Verification items for the finished model (mm, model axes). Face numbers are marked on the shaded views. A direction names the side the tool comes from. Give positions to 0.01 mm unless a question says otherwise; leave off trailing zeros. Loops run counter-clockwise (first coordinate to the right, second up) from the corner with the lowest first, then second, coordinate; pieces in that order, holes last. Notation, with made-up numbers: M 69.25,-26 L 92.25,-26 A29 ccw 92.25,-5 Z; hole C 83.25,-38 d6. An arc over 180 degrees is marked long. Put each result on its own line as item: value. Start each with the question number.
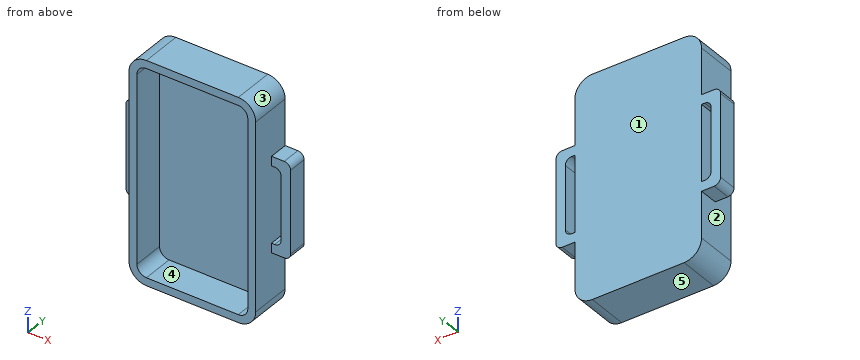
from build123d import *

# Parameters (mm, degrees)
F1_DEPTH = 3
F2_DEPTH = 13
F3_DEPTH = 6


with BuildPart() as f1:
    # F0 (on Front) → F1 (new body)
    with BuildSketch(Plane.XZ):
        with BuildLine():
            Line((-14.5, -32.5), (14.5, -32.5))
            ThreePointArc((14.5, -32.5), (16.62132, -31.62132), (17.5, -29.5))
            Line((17.5, -29.5), (17.5, 29.5))
            ThreePointArc((17.5, 29.5), (16.62132, 31.62132), (14.5, 32.5))
            Line((14.5, 32.5), (-14.5, 32.5))
            ThreePointArc((-14.5, 32.5), (-16.62132, 31.62132), (-17.5, 29.5))
            Line((-17.5, 29.5), (-17.5, -29.5))
            ThreePointArc((-17.5, -29.5), (-16.62132, -31.62132), (-14.5, -32.5))
        make_face()
    extrude(amount=F1_DEPTH)

    # F0 (on Front) → F2 (join)
    with BuildSketch(Plane.XZ):
        with BuildLine():
            Line((14.5, 35), (-14.5, 35))
            ThreePointArc((-14.5, 35), (-18.389087, 33.389087), (-20, 29.5))
            Line((-20, 29.5), (-20, 15))
            Line((-20, 15), (-20, 12))
            Line((-20, 12), (-20, -12))
            Line((-20, -12), (-20, -15))
            Line((-20, -15), (-20, -29.5))
            ThreePointArc((-20, -29.5), (-18.389087, -33.389087), (-14.5, -35))
            Line((-14.5, -35), (14.5, -35))
            ThreePointArc((14.5, -35), (18.389087, -33.389087), (20, -29.5))
            Line((20, -29.5), (20, -15))
            Line((20, -15), (20, -12))
            Line((20, -12), (20, 12))
            Line((20, 12), (20, 15))
            Line((20, 15), (20, 29.5))
            ThreePointArc((20, 29.5), (18.389087, 33.389087), (14.5, 35))
        make_face()
        with BuildLine():
            ThreePointArc((17.5, -29.5), (16.62132, -31.62132), (14.5, -32.5))
            Line((14.5, -32.5), (-14.5, -32.5))
            ThreePointArc((-14.5, -32.5), (-16.62132, -31.62132), (-17.5, -29.5))
            Line((-17.5, -29.5), (-17.5, 29.5))
            ThreePointArc((-17.5, 29.5), (-16.62132, 31.62132), (-14.5, 32.5))
            Line((-14.5, 32.5), (14.5, 32.5))
            ThreePointArc((14.5, 32.5), (16.62132, 31.62132), (17.5, 29.5))
            Line((17.5, 29.5), (17.5, -29.5))
        make_face(mode=Mode.SUBTRACT)
    extrude(amount=F2_DEPTH)

    # F0 (on Front) → F3 (join)
    with BuildSketch(Plane.XZ):
        with BuildLine():
            Line((-20, 12), (-20, 15))
            Line((-20, 15), (-24, 15))
            ThreePointArc((-24, 15), (-25.414214, 14.414214), (-26, 13))
            Line((-26, 13), (-26, -13))
            ThreePointArc((-26, -13), (-25.414214, -14.414214), (-24, -15))
            Line((-24, -15), (-20, -15))
            Line((-20, -15), (-20, -12))
            Line((-20, -12), (-21, -12))
            ThreePointArc((-21, -12), (-22.414214, -11.414214), (-23, -10))
            Line((-23, -10), (-23, 10))
            ThreePointArc((-23, 10), (-22.414214, 11.414214), (-21, 12))
            Line((-21, 12), (-20, 12))
        make_face()
        with BuildLine():
            Line((24, 15), (20, 15))
            Line((20, 15), (20, 12))
            Line((20, 12), (21, 12))
            ThreePointArc((21, 12), (22.414214, 11.414214), (23, 10))
            Line((23, 10), (23, -10))
            ThreePointArc((23, -10), (22.414214, -11.414214), (21, -12))
            Line((21, -12), (20, -12))
            Line((20, -12), (20, -15))
            Line((20, -15), (24, -15))
            ThreePointArc((24, -15), (25.414214, -14.414214), (26, -13))
            Line((26, -13), (26, 13))
            ThreePointArc((26, 13), (25.414214, 14.414214), (24, 15))
        make_face()
    extrude(amount=F3_DEPTH)


solid = f1.part
Q1. Cross-section at B-B, the plane y = -10. Record the boundary of the cut face in (x, z).
Q2. Go/stop test with flat-tipped pins: pin 1 (0.5 mm diameter, centred on x = 20.5, y = -3, fed in from +Z); pin 2 (1 mm diameter, centred on y = -4.5, z = -17.5, fed in from +X); pin 3 (3 mm diameter, centred on x = 22.5, z = -2.5, fed in from -Y); pin 4 (5 mm diameter, centred on x = -21.5, z = -2.5, fed in from -Y). Record where each tip stops, or that it passes through.
Q3. Cross-section at C-C, the plane x = 4. Record the boundary of the cut face in (y, z), then the cut area to 3 significant figures.
Q4. Cross-section at D-D, the plane z = 17. Record the boundary of the cut face in (x, y).
Q5. Cross-section at A-A, the plane z = 4. Record the boundary of the cut face in (x, y), then the cut area to 3 significant figures.
Q6. Scan lines: L1, parallel to X at y = -1, z = -1; L2, parallel to Z at x = -9.5, y = -3.5; L3, parallel to X at y = -10.25, z = -12. Record each from-to range of solid material in increasing order.
Q7. Release check for a two-part mould opening along Z. For the marked faces 3, 4 and 5 record: pulls with the +Z half, pulls with the -Z half, needs draft (parallel to the pull), parting line crosses it, or undercut.
Q8. Set-up check for the marked faces 1 and 2: record each of +Z, -Z, +X, -X, +Y, -Y from which the full face is reachable in a straight line by a thin tool's end or side.
Ans:
1. outline: M -20,-29.5 A5.5 ccw -14.5,-35 L 14.5,-35 A5.5 ccw 20,-29.5 L 20,29.5 A5.5 ccw 14.5,35 L -14.5,35 A5.5 ccw -20,29.5 Z; hole M -17.5,-29.5 A3 ccw -14.5,-32.5 L 14.5,-32.5 A3 ccw 17.5,-29.5 L 17.5,29.5 A3 ccw 14.5,32.5 L -14.5,32.5 A3 ccw -17.5,29.5 Z
2. pin 1: stops at z = 15
2. pin 2: stops at x = 20
2. pin 3: stops at y = -6
2. pin 4: stops at y = -13
3. outline: M -13,-35 L 0,-35 L 0,35 L -13,35 L -13,32.5 L -3,32.5 L -3,-32.5 L -13,-32.5 Z
3. area: 260 mm^2
4. outline: M -20,-13 L -17.5,-13 L -17.5,-3 L 17.5,-3 L 17.5,-13 L 20,-13 L 20,0 L -20,0 Z
5. outline: M -26,-6 L -23,-6 L -23,0 L -26,0 Z; M -20,-13 L -17.5,-13 L -17.5,-3 L 17.5,-3 L 17.5,-13 L 20,-13 L 20,0 L -20,0 Z; M 23,-6 L 26,-6 L 26,0 L 23,0 Z
5. area: 206 mm^2
6. L1: x = -26 to -23, -20 to 20, 23 to 26
6. L2: z = -35 to -32.5, 32.5 to 35
6. L3: x = -20 to -17.5, 17.5 to 20
7. face 3: pulls with the +Z half
7. face 4: undercut
7. face 5: pulls with the -Z half
8. face 1: +Z, -Z, +X, -X, +Y
8. face 2: -Y
